Could you check a few things on this model? Use its own coordinates, in mm. A direction names the side the tool comes from. Round coordinates to 2 decimals unless told otherwise and drop trailing zeros. Loops run counter-clockwise (first coordinate to the right, second up) from the corner with the lowest first, then second, coordinate; pieces in that order, holes last.
from build123d import *

# Parameters (mm, degrees)
F0_W      = 63.8
F0_H      = 31.8
F0_W_2    = 60.8
F0_H_2    = 28.8
F1_DEPTH  = 12.8
F2_W      = 6.3
F2_H      = 6.3
F2_W_2    = 7.8
F3_DEPTH  = 1
F4_R      = 2.45
F5_DEPTH  = 1.8
F6_W      = 0.85
F6_H      = 0.5
F7_DEPTH  = 25.4
F9_DEPTH  = 8
F11_DEPTH = 5
F12_W     = 0.1
F12_H     = 1
F13_DEPTH = 6.3
F14_W     = 6
F14_H     = 1.7
F15_DEPTH = 2.54
F16_W     = 11
F16_H     = 6
F16_W_2   = 6
F16_H_2   = 1.7
F17_DEPTH = 0.5
F19_DEPTH = 5
F21_DEPTH = 4
F22_W     = 6.096
F22_H     = 6.096
F23_DEPTH = 25.4
F24_W     = 1.0284033013
F24_H     = 6.0595651898
F25_DEPTH = 3.81
F26_W     = 1.0230291676
F26_H     = 6.1809321209
F27_DEPTH = 3.81
F28_W     = 8.1515833735
F28_H     = 1.3899055775
F29_DEPTH = 3.81


# Not quite as in the source:
# - a feature names something its author has since deleted; it is built from what else it names


with BuildPart() as f1:
    # F0 (on Top) → F1 (new body)
    with BuildSketch(Plane.XY):
        with Locations((31.9, 15.9)):
            Rectangle(F0_W, F0_H)
        with Locations((31.9, 15.9)):
            Rectangle(F0_W_2, F0_H_2, mode=Mode.SUBTRACT)
    extrude(amount=F1_DEPTH)

    # F2 (on face) → F3 (join)
    with BuildSketch(Plane.XY.offset(12.8)):
        with Locations((4.65, 27.15)):
            Rectangle(F2_W, F2_H)
        with Locations((4.65, 4.65)):
            Rectangle(F2_W, F2_H)
        with Locations((59.15, 4.65)):
            Rectangle(F2_W, F2_H)
        with Locations((59.15, 27.15)):
            Rectangle(F2_W, F2_H)
        with Locations((27.9, 27.15)):
            Rectangle(F2_W_2, F2_H)
        with Locations((35.9, 4.65)):
            Rectangle(F2_W_2, F2_H)
    extrude(amount=-F3_DEPTH)

    # F4 (on face) → F5 (join)
    with BuildSketch(Plane.XY.offset(12.8)):
        with Locations((3.9, 27.9)):
            Circle(F4_R)
        with Locations((59.9, 27.9)):
            Circle(F4_R)
        with Locations((59.9, 3.9)):
            Circle(F4_R)
        with Locations((3.9, 3.9)):
            Circle(F4_R)
        with Locations((27.9, 27.9)):
            Circle(F4_R)
        with Locations((35.9, 3.9)):
            Circle(F4_R)
    extrude(amount=F5_DEPTH)

    # F6 (on face) → F7 (cut)
    with BuildSketch(Plane.XZ):
        Polygon((11.575, 10.95), (9.7, 10.95), (9.7, 7.15), (14.3, 7.15), (14.3, 10.95), (12.425, 10.95), align=None)
        with Locations((12, 11.2)):
            Rectangle(F6_W, F6_H)
    extrude(amount=-F7_DEPTH, mode=Mode.SUBTRACT)

    # F8 (on face) → F9 (join)
    with BuildSketch(Plane(origin=(0, 1.5, 0), x_dir=(-1, 0, 0), z_dir=(0, 1, 0))):
        Polygon((-13.6, 5.8), (-13.6, 6.8), (-15.1, 6.8), (-15.1, 11.8), (-13.6, 11.8), (-13.6, 12.8), (-16.1, 12.8), (-16.1, 5.8), align=None)
        Polygon((-8.9, 6.8), (-10.4, 6.8), (-10.4, 5.8), (-7.9, 5.8), (-7.9, 12.8), (-10.4, 12.8), (-10.4, 11.8), (-8.9, 11.8), align=None)
    extrude(amount=F9_DEPTH)

    # F10 (on face) → F11 (join, through all)
    with BuildSketch(Plane.XY.offset(6.8)):
        Polygon((14.6, 7.6), (15.1, 7.6), (15.1, 9.5), align=None)
        Polygon((9.4, 7.6), (8.9, 9.5), (8.9, 7.6), align=None)
    extrude(amount=F11_DEPTH)

    # F12 (on face) → F13 (join, through all)
    with BuildSketch(Plane(origin=(0, 1.5, 0), x_dir=(-1, 0, 0), z_dir=(0, 1, 0))):
        with Locations((-7.85, 12.3)):
            Rectangle(F12_W, F12_H)
    extrude(amount=F13_DEPTH)

    # F14 (on face) → F15 (cut)
    with BuildSketch(Plane(origin=(0, 31.8, 0), x_dir=(-1, 0, 0), z_dir=(0, 1, 0))):
        with Locations((-12, 6.4)):
            Rectangle(F14_W, F14_H)
    extrude(amount=-F15_DEPTH, mode=Mode.SUBTRACT)

    # F16 (on face) → F17 (join)
    with BuildSketch(Plane.XZ.offset(-30.3)):
        with Locations((12, 6.4)):
            Rectangle(F16_W, F16_H)
        with Locations((12, 6.4)):
            Rectangle(F16_W_2, F16_H_2, mode=Mode.SUBTRACT)
    extrude(amount=F17_DEPTH)

    # F18 (on face) → F19 (join)
    with BuildSketch(Plane.XZ.offset(-29.8)):
        Polygon((9, 9.4), (6.5, 9.4), (6.5, 3.4), (9, 3.4), (9, 4.4), (7.5, 4.4), (7.5, 8.4), (9, 8.4), align=None)
        Polygon((17.5, 9.4), (15, 9.4), (15, 8.4), (16.5, 8.4), (16.5, 4.4), (15, 4.4), (15, 3.4), (17.5, 3.4), align=None)
    extrude(amount=F19_DEPTH)

    # F20 (on face) → F21 (join, through all)
    with BuildSketch(Plane.XY.offset(4.4)):
        Polygon((7.5, 25.8), (7.5, 24.8), (8, 25.8), align=None)
        Polygon((16, 25.8), (16.5, 24.8), (16.5, 25.8), align=None)
    extrude(amount=F21_DEPTH)

    # F22 (on face) → F23 (cut)
    with BuildSketch(Plane(origin=(0, 0, 0), x_dir=(0, -1, 0), z_dir=(-1, 0, 0))):
        with Locations((-16.5878270902, 6.4446975011)):
            Rectangle(F22_W, F22_H)
    extrude(amount=-F23_DEPTH, mode=Mode.SUBTRACT)

    # F24 (on face) → F25 (join)
    with BuildSketch(Plane.YZ.offset(1.5)):
        with Locations((13.0256254396, 6.4629149062)):
            Rectangle(F24_W, F24_H)
    extrude(amount=F25_DEPTH)

    # F26 (on face) → F27 (join)
    with BuildSketch(Plane.YZ.offset(1.5)):
        with Locations((20.147341674, 6.4022314407)):
            Rectangle(F26_W, F26_H)
    extrude(amount=F27_DEPTH)

    # F28 (on face) → F29 (join)
    with BuildSketch(Plane.YZ.offset(1.5)):
        with Locations((16.583064571, 2.6168125914)):
            Rectangle(F28_W, F28_H)
    extrude(amount=F29_DEPTH)


solid = f1.part
Item 1: If I drill on line 1 along X through (y, z) = (28.5, 7.5); line 2 along X through (y, z) = (5, 11.5); line 3 along X through (y, z) = (4.5, 5.75), over which ranges is the centre line in solid material (lowest first)?
Results list:
line 1: x = 0 to 1.5, 6.5 to 7.5, 16.5 to 17.5, 62.3 to 63.8
line 2: x = 0 to 1.5, 7.9 to 8.9, 15.1 to 16.1, 62.3 to 63.8
line 3: x = 0 to 1.5, 62.3 to 63.8
Item 2: We'd pull the mould along X, two halves only. Please class faces 5 (the flat face through (16.1, 5, 9)), 6 (the flat face through (31, 31.8, 6)): released by +X, released by -X, zero draft, split by the parting line, or undercut.
Results list:
face 5: undercut
face 6: zero draft
Item 3: If we section it at B-B, the plane x = 3.9: Count the separate pieces of the cut face and the enclosed holes in it, then the cut area to 3 significant figures.
Results list:
separate pieces: 4
enclosed holes: 0
area: 92.5 mm2
Item 4: Will these pins go through, and if not, where does the flat tip stop? pin 1 (10 mm diameter, centred on x = 54.5, y = 6.5, fed in from +Z); pin 2 (6 mm diameter, centred on x = 13, y = 26.5, fed in from -Z); pin 3 (10 mm diameter, centred on x = 44.5, y = 11.5, fed in from -Z); pin 4 (3 mm diameter, centred on x = 15.5, y = 4.5, fed in from -Z).
Results list:
pin 1: stops at z = 14.6
pin 2: stops at z = 3.4
pin 3: passes through
pin 4: stops at z = 5.8
Item 5: If we section it at A-A, the plane x = 59.9: Please give me the cut outline in (y, z).
Results list:
outline: (0, 0) - (1.5, 0) - (1.5, 11.8) - (7.8, 11.8) - (7.8, 12.8) - (6.35, 12.8) - (6.35, 14.6) - (1.45, 14.6) - (1.45, 12.8) - (0, 12.8) - close; (24, 11.8) - (30.3, 11.8) - (30.3, 0) - (31.8, 0) - (31.8, 12.8) - (30.35, 12.8) - (30.35, 14.6) - (25.45, 14.6) - (25.45, 12.8) - (24, 12.8) - close
Item 6: For faces 1 (the cylindrical face through (3.4, 1.5, 13.7)), 2 (the flat face through (15, 31, 6)), 3 (the flat face through (7, 24.8, 6)), 4 (the flat face through (8, 27, 4.4)), which set-ups out of +Z, -Z, +X, -X, +Y, -Y let a thin tool reach every point of the face, with its end or its side?
Results list:
face 1: +Z
face 2: +Y
face 3: -Z
face 4: none
